Input: dimensioned drawing with shaded views. Units: mm. Origin: part minimum x, y, z. A direction names the side the tool comes from. Coordinates: 2 decimals unless noted, no trailing zeros. Write each loop counter-clockwise with the first axis right and the second up, starting at its lowest first coordinate (ties: lowest second). Pieces come first, ordered by that corner, then holes. Notation, with made-up numbers: (-27, -5) - (-10, -5) arc R4 cw to (-10, 1) - close; hole circle Ø7 at (64.5, 28). An arc over 180 degrees is marked (long way). One line per question, with ' | ' between items.
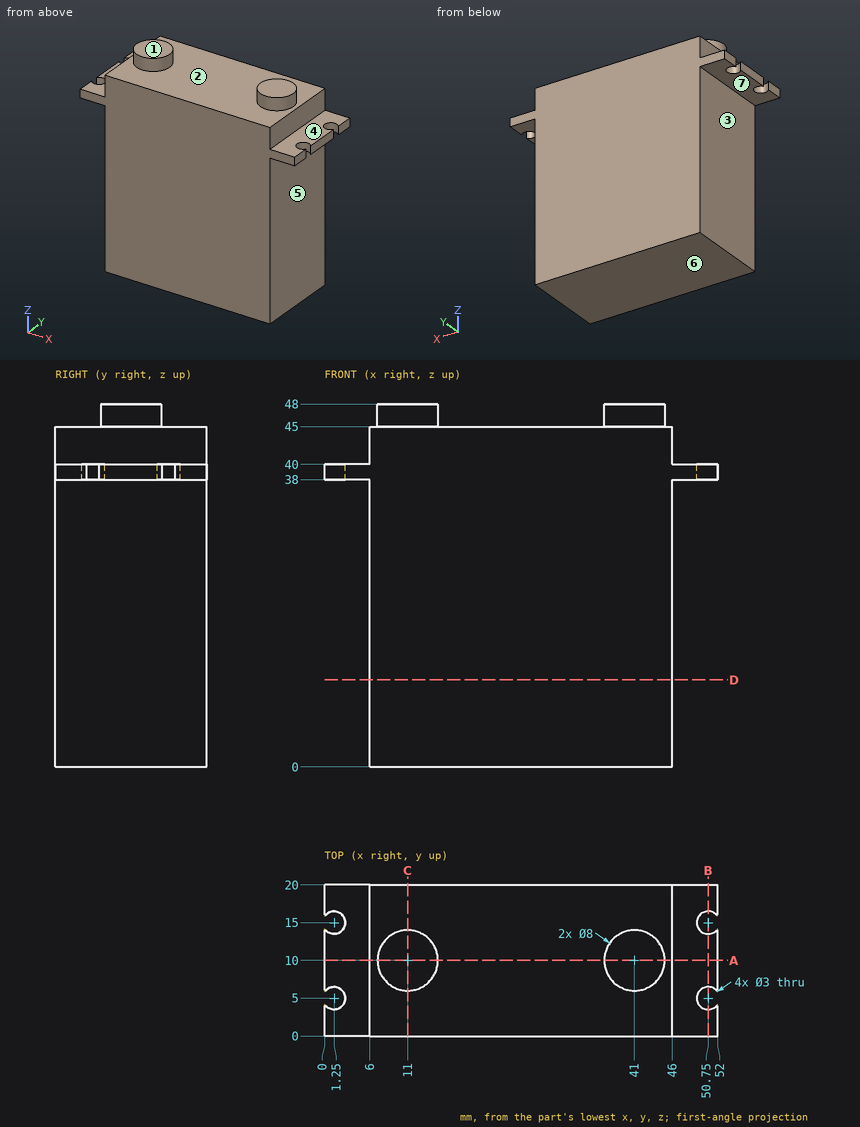
Item 1: Cut plane D-D on z = 11.5. Return loops of the section in (x, y), and give its area (3 significant figures).
Check sheet entries:
outline: (6, 0) - (46, 0) - (46, 20) - (6, 20) - close | area: 800 mm²
Item 2: Mould query, pull axis X, two halves, no side actions, for the marked faces 1, 2 and 3. Classes: pulls with the +X half, pulls with the -X half, needs draft (parallel to the pull), parting line crosses it, or undercut.
Check sheet entries:
face 1: needs draft | face 2: undercut | face 3: pulls with the -X half
Item 3: Cut plane A-A on y = 10. Return loops of the section in (x, z), and give its area (3 significant figures).
Check sheet entries:
outline: (0, 38) - (6, 38) - (6, 0) - (46, 0) - (46, 38) - (52, 38) - (52, 40) - (46, 40) - (46, 45) - (45, 45) - (45, 48) - (37, 48) - (37, 45) - (15, 45) - (15, 48) - (7, 48) - (7, 45) - (6, 45) - (6, 40) - (0, 40) - close | area: 1,870 mm²
Item 4: Access query for the marked faces 4, 5, 6 and 7. Directions: +Z, -Z, +X, -X, +Y, -Y. A direction counts if a zero-diameter tool reaches every point of the face in a straight line with its end or side. Return the directions, or none.
Check sheet entries:
face 4: +Z, +X, +Y, -Y | face 5: -Z, +X, +Y, -Y | face 6: -Z, +X, -X, +Y, -Y | face 7: -Z, -X, +Y, -Y
Item 5: Ray query, line 1 along Y through (x, z) = (1.25, 39.1); line 2 along Y through (x, z) = (50, 39); line 3 along Z through (x, y) = (5, 13). Return the intervals inside material, ascending. Write a range as [from, to].
Check sheet entries:
line 1: [0, 3.5], [6.5, 13.5], [16.5, 20] | line 2: [0, 3.7], [6.3, 13.7], [16.3, 20] | line 3: [38, 40]
Item 6: Cut plane C-C on x = 11. Return loops of the section in (y, z).
Check sheet entries:
outline: (0, 0) - (20, 0) - (20, 45) - (14, 45) - (14, 48) - (6, 48) - (6, 45) - (0, 45) - close
Item 7: Cut plane B-B on x = 50.75. Return loops of the section in (y, z).
Check sheet entries:
outline: (0, 38) - (3.5, 38) - (3.5, 40) - (0, 40) - close; (6.5, 38) - (13.5, 38) - (13.5, 40) - (6.5, 40) - close; (16.5, 38) - (20, 38) - (20, 40) - (16.5, 40) - close
Item 8: Pin query (flat end, axial travel): pin 1 Ø6 at (x, y) = (31, 9.5) entering from +Z; pin 2 Ø6 at (y, z) = (12, 19) entering from +X; pin 3 Ø1 at (y, z) = (16, 35.5) entering from -X. Return the tip coordinate at first contact, or that it passes through.
Check sheet entries:
pin 1: z = 45 | pin 2: x = 46 | pin 3: x = 6
